Model file for the job. Use its own axes, mm. A direction names the side the tool comes from. Round coordinates to 2 decimals unless told otherwise and drop trailing zeros. Loops run counter-clockwise (first coordinate to the right, second up) from the corner with the lowest first, then second, coordinate; pieces in that order, holes last. Notation, with made-up numbers: M 51.25,73 L 100.25,73 A24 cw 100.25,110 Z; hole C 8,42.25 d5. An arc over 180 degrees is marked long. Answer in a Markdown table with one row per item.
from build123d import *

# Parameters (mm, degrees)
SKETCH2_R          = 2.54
CUT_EXTRUDE1_DEPTH = 21.635057548


with BuildPart() as part:
    # Sketch1 → Revolve1 (revolve)
    with BuildSketch(Plane.XY, mode=Mode.PRIVATE) as revolve1_sk:
        with BuildLine():
            Line((0, 0), (0, 10.16))
            Line((0, 10.16), (4.318, 10.16))
            Line((4.318, 10.16), (4.318, 9.398))
            Line((4.318, 9.398), (12.7, 9.398))
            Line((12.7, 9.398), (12.7, 8.128))
            ThreePointArc((12.7, 8.128), (9.652, 5.08), (12.7, 2.032))
            Line((12.7, 2.032), (12.7, 0.762))
            Line((12.7, 0.762), (4.318, 0.762))
            Line((4.318, 0.762), (4.318, 0))
            Line((4.318, 0), (0, 0))
        make_face()
    revolve(revolve1_sk.sketch.rotate(Axis((0, 0, 0), (0, 1, 0)), 90), axis=Axis((0, 0, 0), (0, 1, 0)))

    # Sketch2 → Cut-Extrude1 (cut, through all)
    with BuildSketch(Plane(origin=(0, 10.16, 0), x_dir=(1, 0, 0), z_dir=(0, 1, 0))):
        with Locations(Location((0, 0, 0), (0, 0, 270))):
            Circle(SKETCH2_R)
    extrude(amount=-CUT_EXTRUDE1_DEPTH, mode=Mode.SUBTRACT)


solid = part.part
1. Tool access for faces 4 (the flat face through (0, 0.762, -5)), 5 (the flat face through (2, 0, -2)), 6 (the cylindrical face through (-4.28, 9.77, 0.56)): list every direction of +Z, -Z, +X, -X, +Y, -Y with a clear straight run to the whole face (end or side of a thin tool).
Verdict:
| item | result |
|---|---|
| face 4 | -Y |
| face 5 | +Z, -Z, +X, -X, -Y |
| face 6 | +Y |
2. Saw through at A-A (z = 0). Write the cut outline in (x, y).
Verdict:
| item | result |
|---|---|
| outline | M -12.7,0.76 L -4.32,0.76 L -4.32,0 L -2.54,0 L -2.54,10.16 L -4.32,10.16 L -4.32,9.4 L -12.7,9.4 L -12.7,8.13 A3.05 cw -12.7,2.03 Z; M 2.54,0 L 4.32,0 L 4.32,0.76 L 12.7,0.76 L 12.7,2.03 A3.05 cw 12.7,8.13 L 12.7,9.4 L 4.32,9.4 L 4.32,10.16 L 2.54,10.16 Z |
3. Saw through at B-B (x = 0). Write the cut outline in (y, z), and give its area (3 significant figures).
Verdict:
| item | result |
|---|---|
| outline | M 0,-4.32 L 0.76,-4.32 L 0.76,-12.7 L 2.03,-12.7 A3.05 cw 8.13,-12.7 L 9.4,-12.7 L 9.4,-4.32 L 10.16,-4.32 L 10.16,-2.54 L 0,-2.54 Z; M 0,2.54 L 10.16,2.54 L 10.16,4.32 L 9.4,4.32 L 9.4,12.7 L 8.13,12.7 A3.05 cw 2.03,12.7 L 0.76,12.7 L 0.76,4.32 L 0,4.32 Z |
| area | 152 mm² |
4. Pin check, flat tips, straight feed: pin 1 (12.5 mm diameter, centred on x = 4, z = 5, fed in from +Y); pin 2 (4 mm diameter, centred on x = 7, z = 2, fed in from -Y). Stop position of each tip, or through.
Verdict:
| item | result |
|---|---|
| pin 1 | stops at y = 10.16 |
| pin 2 | stops at y = 0.76 |
5. Wall check: probe 1 along Y at (x, z) = (3.75, -5.75); probe 2 along Y at (x, z) = (10.25, -5); probe 3 along Y at (x, z) = (-9.25, -4.75). Give the ranges that are in metal, low to high.
Verdict:
| item | result |
|---|---|
| probe 1 | y = 0.76 to 9.4 |
| probe 2 | y = 0.76 to 2.32, 7.84 to 9.4 |
| probe 3 | y = 0.76 to 3.08, 7.08 to 9.4 |
6. Mould opens along X. For faces 1 (the flat face through (0, 9.398, 5)), 2 (the cylindrical face through (2.52, 5.15, -0.33)), 3 (the cylindrical face through (-4.28, 0.38, 0.56)) say: +X half, -X half, draft (parallel to the pull), parting line (faces both ways), or undercut.
Verdict:
| item | result |
|---|---|
| face 1 | draft |
| face 2 | undercut |
| face 3 | parting line |
